```python
from build123d import *

# Parameters (mm, degrees)
SKETCH_1_W          = 56
SKETCH_1_H          = 38
EXTRUDE_1_DEPTH     = 10
SKETCH_2_W          = 15
SKETCH_2_H          = 13.2
SKETCH_2_W_2        = 1.48
SKETCH_2_H_2        = 2.27
CUT_EXTRUDE_1_DEPTH = 8
SKETCH_3_W          = 53.7
SKETCH_3_H          = 22.7
CUT_EXTRUDE_2_DEPTH = 2
CUT_EXTRUDE_4_REACH = 61.975
SKETCH_5_W          = 3.2
SKETCH_5_H          = 8.5
CUT_EXTRUDE_5_REACH = 61.975
SKETCH_6_W          = 3.8
SKETCH_6_H          = 12
SKETCH_7_R          = 1.6
CUT_EXTRUDE_6_DEPTH = 36.284557529
FILLET_1_R          = 2
CUT_EXTRUDE_7_DEPTH = 5
FILLET_3_R          = 2
FILLET_4_R          = 1
SKETCH_10_W         = 53.7
SKETCH_10_H         = 18
CUT_EXTRUDE_9_DEPTH = 4


with BuildPart() as part:
    # 草图1 → 凸台-拉伸1 (new body)
    with BuildSketch(Plane.XY):
        Rectangle(SKETCH_1_W, SKETCH_1_H)
    extrude(amount=EXTRUDE_1_DEPTH)

    # 草图2 → 切除-拉伸1 (cut)
    with BuildSketch(Plane.XY.offset(10)):
        with Locations((-13.5, 0)):
            Rectangle(SKETCH_2_W, SKETCH_2_H)
        with Locations((17.09, 3.515)):
            Rectangle(SKETCH_2_W_2, SKETCH_2_H_2)
        with Locations((17.09, -2.975)):
            Rectangle(SKETCH_2_W_2, SKETCH_2_H_2)
    extrude(amount=-CUT_EXTRUDE_1_DEPTH, mode=Mode.SUBTRACT)

    # 草图3 → 切除-拉伸2 (cut)
    with BuildSketch(Plane(origin=(0, 0, 0), x_dir=(-1, 0, 0), z_dir=(0, 0, -1))):
        Rectangle(SKETCH_3_W, SKETCH_3_H)
    extrude(amount=-CUT_EXTRUDE_2_DEPTH, mode=Mode.SUBTRACT)

    # 草图5 → 切除-拉伸4 (cut, up to next)
    with BuildSketch(Plane.ZY.offset(28), mode=Mode.PRIVATE) as cut_extrude_4_sk1:
        with Locations((3.18, 0)):
            Rectangle(SKETCH_5_W, SKETCH_5_H)
    cut_extrude_4_tool1 = extrude(cut_extrude_4_sk1.sketch, amount=-CUT_EXTRUDE_4_REACH, mode=Mode.PRIVATE) & part.part
    add(cut_extrude_4_tool1.solids().sort_by_distance((-28, 0, 3.18))[0], mode=Mode.SUBTRACT)

    # 草图6 → 切除-拉伸5 (cut, up to next)
    with BuildSketch(Plane(origin=(28, 0, 0), x_dir=(0, 0, -1), z_dir=(1, 0, 0)), mode=Mode.PRIVATE) as cut_extrude_5_sk1:
        with Locations((-3.7, 0)):
            Rectangle(SKETCH_6_W, SKETCH_6_H)
    cut_extrude_5_tool1 = extrude(cut_extrude_5_sk1.sketch, amount=-CUT_EXTRUDE_5_REACH, mode=Mode.PRIVATE) & part.part
    add(cut_extrude_5_tool1.solids().sort_by_distance((28, 0, 3.7))[0], mode=Mode.SUBTRACT)

    # 草图7 → 切除-拉伸6 (cut, through all)
    with BuildSketch(Plane(origin=(0, 0, 0), x_dir=(-1, 0, 0), z_dir=(0, 0, -1))):
        with Locations((25.5, 16)):
            Circle(SKETCH_7_R)
        with Locations(Location((25.5, -16, 0), (0, 0, 180))):
            Circle(SKETCH_7_R)
        with Locations((-25.5, -16)):
            Circle(SKETCH_7_R)
        with Locations(Location((-25.5, 16, 0), (0, 0, 180))):
            Circle(SKETCH_7_R)
    extrude(amount=-CUT_EXTRUDE_6_DEPTH, mode=Mode.SUBTRACT)

    # 圆角1
    fillet_1_edges = [part.edges().sort_by_distance(p)[0] for p in [
        (28, -19, 5),
        (-28, -19, 5),
        (-28, 19, 5),
        (28, 19, 5),
    ]]
    fillet(fillet_1_edges, radius=FILLET_1_R)

    # 草图8 → 切除-拉伸7 (cut)
    with BuildSketch(Plane.XY.offset(10)):
        with BuildLine():
            Line((-22.3, 16), (-22.3, 19))
            Line((-22.3, 19), (-26, 19))
            ThreePointArc((-26, 19), (-27.414213562, 18.414213562), (-28, 17))
            Line((-28, 17), (-28, 12.8))
            Line((-28, 12.8), (-25.5, 12.8))
            ThreePointArc((-25.5, 12.8), (-23.2372583, 13.7372583), (-22.3, 16))
        make_face()
        with BuildLine():
            Line((28, 12.8), (28, 17))
            ThreePointArc((28, 17), (27.414213562, 18.414213562), (26, 19))
            Line((26, 19), (22.3, 19))
            Line((22.3, 19), (22.3, 16))
            ThreePointArc((22.3, 16), (23.2372583, 13.7372583), (25.5, 12.8))
            Line((25.5, 12.8), (28, 12.8))
        make_face()
        with BuildLine():
            Line((-28, -12.8), (-28, -17))
            ThreePointArc((-28, -17), (-27.414213562, -18.414213562), (-26, -19))
            Line((-26, -19), (-22.3, -19))
            Line((-22.3, -19), (-22.3, -16))
            ThreePointArc((-22.3, -16), (-23.2372583, -13.7372583), (-25.5, -12.8))
            Line((-25.5, -12.8), (-28, -12.8))
        make_face()
        with BuildLine():
            Line((26, -19), (22.3, -19))
            Line((22.3, -19), (22.3, -16))
            ThreePointArc((22.3, -16), (23.2372583, -13.7372583), (25.5, -12.8))
            Line((25.5, -12.8), (28, -12.8))
            Line((28, -12.8), (28, -17))
            ThreePointArc((28, -17), (27.414213562, -18.414213562), (26, -19))
        make_face()
    extrude(amount=-CUT_EXTRUDE_7_DEPTH, mode=Mode.SUBTRACT)

    # 圆角3
    fillet_3_edges = [part.edges().sort_by_distance(p)[0] for p in [
        (28, 12.8, 7.5),
        (22.3, 19, 7.5),
        (-28, -12.8, 7.5),
        (-22.3, -19, 7.5),
        (22.3, -19, 7.5),
        (28, -12.8, 7.5),
        (-28, 12.8, 7.5),
        (-22.3, 19, 7.5),
    ]]
    fillet(fillet_3_edges, radius=FILLET_3_R)

    # 圆角4
    fillet_4_edges = [part.edges().sort_by_distance(p)[0] for p in [
        (23.2372583, 13.7372583, 10),
        (25.75, 12.8, 10),
        (-23.2372583, -13.7372583, 10),
        (-25.75, -12.8, 10),
        (-6, 0, 10),
        (23.2372583, -13.7372583, 10),
        (-13.5, 6.6, 10),
        (22.3, -16.5, 10),
        (-21, 0, 10),
        (-13.5, -6.6, 10),
        (-23.2372583, 13.7372583, 10),
        (-22.3, 16.5, 10),
        (0, -19, 10),
        (28, 0, 10),
        (22.3, 16.5, 10),
        (0, 19, 10),
        (-25.75, 12.8, 10),
        (-28, 0, 10),
        (-22.3, -16.5, 10),
        (25.75, -12.8, 10),
        (-27.414213562, -12.214213562, 10),
        (-21.714213562, -18.414213562, 10),
        (-27.414213562, 12.214213562, 10),
        (-21.714213562, 18.414213562, 10),
        (27.414213562, 12.214213562, 10),
        (21.714213562, 18.414213562, 10),
        (27.414213562, -12.214213562, 10),
        (21.714213562, -18.414213562, 10),
    ]]
    fillet(fillet_4_edges, radius=FILLET_4_R)

    # 草图10 → 切除-拉伸9 (cut)
    with BuildSketch(Plane(origin=(0, 0, 0), x_dir=(-1, 0, 0), z_dir=(0, 0, -1))):
        Rectangle(SKETCH_10_W, SKETCH_10_H)
    extrude(amount=-CUT_EXTRUDE_9_DEPTH, mode=Mode.SUBTRACT)


solid = part.part
```
The model under review builds one solid part; all positions refer to its coordinate system, in mm. A direction names the side the tool comes from. Coordinates: 2 decimals unless noted, no trailing zeros. Write each loop counter-clockwise with the first axis right and the second up, starting at its lowest first coordinate (ties: lowest second). Pieces come first, ordered by that corner, then holes.
1) Machinability: for faces 5 (the face through (24, -15, 5)), 6 (the face through (-21, 0, 7)), 7 (the face through (-21.7, 18.43, 6.97)), 8 (the face through (0, -7, 4)), which of the approach directions +Z, -Z, +X, -X, +Y, -Y give a long, thin tool a straight path to every point of the face, cutting with its end or side? Answer none if there is none.
2) We need section D-D on z = 6.25. Count the separate pieces of the cut face and the enclosed holes in it, then the cut area to 3 significant figures.
3) To check wall thickness, follow probe 1 along Y at (x, z) = (-25.5, 2.3); probe 2 along Y at (x, z) = (25.5, 1.05); probe 3 along Y at (x, z) = (-6.5, 1.25). State the ranges of each line that lie inside material, in increasing order.
4) We need section B-B on y = -5. State the section outline as (x, z) points.
5) The part is to be moulded in two halves that separate along X. For faces 1 (the face through (-14, 6.6, 7)), 2 (the face through (-21.7, -18.43, 6.97)), 3 (the face through (23, 14, 7)), 4 (the face through (17.83, 3, 8)), say which applies: pulls with the +X half, pulls with the -X half, needs draft (parallel to the pull), parting line crosses it, or undercut.
6) We need section A-A on y = 3. State the section outline as (x, z) points.
7) Clearance check with flat-ended pins moving along their axes: pin 1 Ø1.5 at (y, z) = (5, 4.5) entering from +X; pin 2 Ø4 at (x, y) = (-3, 8) entering from -Z; pin 3 Ø3 at (x, y) = (25.5, -16) entering from +Z; pin 4 Ø1.2 at (y, z) = (5, 3) entering from +X. State where each tip first meets the part, or that it passes through.
8) We need section C-C on x = -4. State the section outline as (y, z) points, then the cut area to 3 significant figures.
Answer list:
1. face 5: +Z, +X, -Y
1. face 6: +Z, -Z
1. face 7: +Z, -X, +Y
1. face 8: -Z
2. separate pieces: 1
2. enclosed holes: 3
2. area: 1,780 mm2
3. probe 1: y = -19 to -17.6, -14.4 to -9, 9 to 14.4, 17.6 to 19
3. probe 2: y = -19 to -17.6, -14.4 to -11.35, 11.35 to 14.4, 17.6 to 19
3. probe 3: y = -19 to -11.35, 11.35 to 19
4. outline: (-28, 0) - (-26.85, 0) - (-26.85, 4) - (-21, 4) - (-21, 9) arc R1 ccw to (-22, 10) - (-27, 10) arc R1 ccw to (-28, 9) - close; (-6, 5.6) - (28, 5.6) - (28, 9) arc R1 ccw to (27, 10) - (-5, 10) arc R1 ccw to (-6, 9) - close; (26.85, 0) - (28, 0) - (28, 1.8) - (26.85, 1.8) - close
5. face 1: undercut
5. face 2: pulls with the -X half
5. face 3: pulls with the +X half
5. face 4: undercut
6. outline: (-28, 0) - (-26.85, 0) - (-26.85, 1.58) - (-28, 1.58) - close; (-28, 4.78) - (-21, 4.78) - (-21, 9) arc R1 ccw to (-22, 10) - (-27, 10) arc R1 ccw to (-28, 9) - close; (-6, 5.6) - (16.35, 5.6) - (16.35, 10) - (-5, 10) arc R1 ccw to (-6, 9) - close; (17.83, 5.6) - (28, 5.6) - (28, 9) arc R1 ccw to (27, 10) - (17.83, 10) - close; (26.85, 0) - (28, 0) - (28, 1.8) - (26.85, 1.8) - close
7. pin 1: stops at x = -21
7. pin 2: stops at z = 2
7. pin 3: passes through
7. pin 4: stops at x = -26.85
8. outline: (-19, 0) - (-11.35, 0) - (-11.35, 2) - (-9, 2) - (-9, 4) - (-6, 4) - (-6, 5.6) - (6, 5.6) - (6, 4) - (9, 4) - (9, 2) - (11.35, 2) - (11.35, 0) - (19, 0) - (19, 9) arc R1 ccw to (18, 10) - (-18, 10) arc R1 ccw to (-19, 9) - close
8. area: 279 mm2
